from build123d import *

# Parameters (mm, degrees)
F1_DEPTH = 10
F0_R     = 10
F2_DEPTH = 4


with BuildPart() as f1:
    # F0 (on Front) → F1 (new body)
    with BuildSketch(Plane.XZ):
        with BuildLine():
            Line((-19.661892, -15), (-19.661892, 0))
            ThreePointArc((-19.661892, 0), (-16.189862, 11.156988), (-7, 18.373622))
            Line((-7, 18.373622), (-7, 22.602768))
            ThreePointArc((-7, 22.602768), (-19.046238, 14.040155), (-23.661892, 0))
            Line((-23.661892, 0), (-23.661892, -15))
            ThreePointArc((-23.661892, -15), (0, -38.661892), (23.661892, -15))
            Line((23.661892, -15), (23.661892, 0))
            ThreePointArc((23.661892, 0), (20.617598, 11.610331), (12.268062, 20.233136))
            ThreePointArc((12.268062, 20.233136), (9.697053, 21.583612), (6.979972, 22.608961))
            Line((6.979972, 22.608961), (6.979972, 18.38124))
            ThreePointArc((6.979972, 18.38124), (16.18378, 11.165808), (19.661892, 0))
            Line((19.661892, 0), (19.661892, -15))
            ThreePointArc((19.661892, -15), (0, -34.661892), (-19.661892, -15))
        make_face()
    extrude(amount=F1_DEPTH)

    # F0 (on Front) → F2 (join)
    with BuildSketch(Plane.XZ):
        with BuildLine():
            Line((-19.661892, -15), (-19.661892, 0))
            ThreePointArc((-19.661892, 0), (-16.189862, 11.156988), (-7, 18.373622))
            Line((-7, 18.373622), (-7, 22.602768))
            ThreePointArc((-7, 22.602768), (-19.046238, 14.040155), (-23.661892, 0))
            Line((-23.661892, 0), (-23.661892, -15))
            ThreePointArc((-23.661892, -15), (0, -38.661892), (23.661892, -15))
            Line((23.661892, -15), (23.661892, 0))
            ThreePointArc((23.661892, 0), (20.617598, 11.610331), (12.268062, 20.233136))
            ThreePointArc((12.268062, 20.233136), (9.697053, 21.583612), (6.979972, 22.608961))
            Line((6.979972, 22.608961), (6.979972, 18.38124))
            ThreePointArc((6.979972, 18.38124), (16.18378, 11.165808), (19.661892, 0))
            Line((19.661892, 0), (19.661892, -15))
            ThreePointArc((19.661892, -15), (0, -34.661892), (-19.661892, -15))
        make_face()
        with BuildLine():
            ThreePointArc((-7, 18.373622), (-16.189862, 11.156988), (-19.661892, 0))
            Line((-19.661892, 0), (-19.661892, -15))
            ThreePointArc((-19.661892, -15), (0, -34.661892), (19.661892, -15))
            Line((19.661892, -15), (19.661892, 0))
            ThreePointArc((19.661892, 0), (16.18378, 11.165808), (6.979972, 18.38124))
            Line((6.979972, 18.38124), (6.979972, 22.608961))
            ThreePointArc((6.979972, 22.608961), (-0.010482, 23.66189), (-7, 22.602768))
            Line((-7, 22.602768), (-7, 18.373622))
        make_face()
        Circle(F0_R, mode=Mode.SUBTRACT)
        Circle(F0_R)
    extrude(amount=-F2_DEPTH)


solid = f1.part
Read the model definition and answer for the solid it produces. Units are mm, in the model's axes. A direction names the side the tool comes from. Give positions to 0.01 mm unless a question says otherwise; leave off trailing zeros. Loops run counter-clockwise (first coordinate to the right, second up) from the corner with the lowest first, then second, coordinate; pieces in that order, holes last. Notation, with made-up numbers: (21, -35) - (74, -35) arc R25 ccw to (74, 2) - close; hole circle Ø7 at (14, 78.25). An arc over 180 degrees is marked (long way). Answer as CSV lines item,"result". Start each with the question number.
1) Find section B-B (z = -1). Write down the section's boundary in (x, y), then the cut area to 3 significant figures.
2) Find section C-C (x = -11). Write down the section's boundary in (y, z).
3) Find section D-D (y = -5.25). Write down the section's boundary in (x, z).
4) Each of these flat-tipped pins is pushed along its axis until it touches: pin 1 Ø2 at (y, z) = (-6.5, 20.5) entering from +X; pin 2 Ø4 at (y, z) = (1.5, -20.5) entering from -X; pin 3 Ø19.5 at (x, z) = (4, -16.5) entering from -Y. Where does it stop, or does it pass through?
5) Determine the mould class of faces 1 (the face through (9.73, -3.1, 21.57)), 2 (the face through (-16.284, -4.93, 11.02)), 3 (the face through (0, 4, -7)) for opening direction X: released by +X, released by -X, zero draft, split by the parting line, or undercut.
6) Find section A-A (y = 1.25). Write down the section's boundary in (x, z).
7) Which of the six approach directions +Z, -Z, +X, -X, +Y, -Y give full straight-line access (tool end or side, diameter ignored) to faces 4 (the face through (-0.52, -3.098, -38.656)), 5 (the face through (16.09, -4.93, 11.3)), 6 (the face through (-7, -5, 20))?
8) Straight lines are drawn through the part: L1, parallel to X at y = -5.75, z = -6; L2, parallel to Y at x = 4.5, z = -11; L3, parallel to Z at x = 11, y = -5. For each, find the intervals that lie inside material, in ascending order. Write a range as from..to.
Findings below:
1,outline,"(-23.66, -10) - (-19.66, -10) - (-19.66, 0) - (19.66, 0) - (19.66, -10) - (23.66, -10) - (23.66, 4) - (-23.66, 4) - close"
1,area,"269 mm^2"
2,outline,"(-10, -35.95) - (4, -35.95) - (4, 20.95) - (-10, 20.95) - (-10, 16.3) - (0, 16.3) - (0, -31.3) - (-10, -31.3) - close"
3,outline,"(-23.66, -15) arc R23.66 ccw to (23.66, -15) - (23.66, 0) arc R23.66 ccw to (12.27, 20.23) arc R23.66 ccw to (6.98, 22.61) - (6.98, 18.38) arc R19.66 cw to (19.66, 0) - (19.66, -15) arc R19.66 cw to (-19.66, -15) - (-19.66, 0) arc R19.66 cw to (-7, 18.37) - (-7, 22.6) arc R23.66 ccw to (-23.66, 0) - close"
4,pin 1,"x = 13.4"
4,pin 2,"x = -23.4"
4,pin 3,"y = 0"
5,face 1,"released by +X"
5,face 2,"undercut"
5,face 3,"zero draft"
6,outline,"(-23.66, -15) arc R23.66 ccw to (23.66, -15) - (23.66, 0) arc R23.66 ccw to (12.27, 20.23) arc R23.66 ccw to (6.98, 22.61) arc R23.66 ccw to (-7, 22.6) arc R23.66 ccw to (-23.66, 0) - close"
7,face 4,"-Z, +Y, -Y"
7,face 5,"-Y"
7,face 6,"+Z, -Y"
8,L1,"-23.66..-19.66, 19.66..23.66"
8,L2,"0..4"
8,L3,"-35.95..-31.3, 16.3..20.95"
